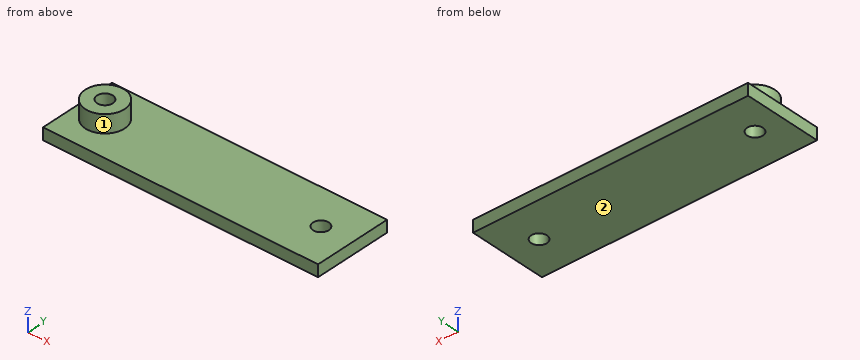
from build123d import *

# Parameters (mm, degrees)
SKETCH1_W           = 70
SKETCH1_H           = 20
BOSS_EXTRUDE1_DEPTH = 3
SKETCH2_R           = 2
CUT_EXTRUDE2_DEPTH  = 37.523964735
SKETCH3_R           = 5
BOSS_EXTRUDE2_DEPTH = 4.5
SKETCH4_R           = 2
CUT_EXTRUDE3_DEPTH  = 4.5


with BuildPart() as part:
    # Sketch1 → Boss-Extrude1 (new body)
    with BuildSketch(Plane.XY):
        Rectangle(SKETCH1_W, SKETCH1_H)
    extrude(amount=BOSS_EXTRUDE1_DEPTH)

    # Sketch2 → Cut-Extrude2 (cut, through all)
    with BuildSketch(Plane.XY.offset(3)):
        with Locations((-28, 0)):
            Circle(SKETCH2_R)
        with Locations((26.96, 0)):
            Circle(SKETCH2_R)
    extrude(amount=-CUT_EXTRUDE2_DEPTH, mode=Mode.SUBTRACT)

    # Sketch3 → Boss-Extrude2 (add)
    with BuildSketch(Plane.XY.offset(3)):
        with Locations((-28, 0)):
            Circle(SKETCH3_R)
    extrude(amount=BOSS_EXTRUDE2_DEPTH)

    # Sketch4 → Cut-Extrude3 (cut)
    with BuildSketch(Plane.XY.offset(7.5)):
        with Locations((-28, 0)):
            Circle(SKETCH4_R)
    extrude(amount=-CUT_EXTRUDE3_DEPTH, mode=Mode.SUBTRACT)


solid = part.part
Model file for the job. Use its own axes, mm. Face numbers are marked on the shaded views. A direction names the side the tool comes from. Coordinates: 2 decimals unless noted, no trailing zeros. Order: outer loops, then holes, each group sorted by start corner. A loop starts at its lowest first (then second) coordinate and runs counter-clockwise, first axis right, second up. Notation, with made-up numbers: (63, 12.25) -> (67, 12.25) arc R12 ccw to (67, 28.25) -> close; hole circle Ø10 at (-32, 29). An arc over 180 degrees is marked (long way). Return JSON: item names as keys, results as strings. Group by question number.
Item 1: Tool access for the marked faces 1 and 2: list every direction of +Z, -Z, +X, -X, +Y, -Y with a clear straight run to the whole face (end or side of a thin tool).
Item 2: Saw through at C-C on y = 0. Write the cut outline in (x, z), then the cut area to 3 significant figures.
Item 3: Saw through at B-B on z = 1.75. Write the cut outline in (x, y).
Item 4: Saw through at A-A on x = 26.96. Write the cut outline in (y, z).
Item 5: Wall check: line 1 along Y through (x, z) = (26.96, 1.85); line 2 along Y through (x, z) = (-28, 4); line 3 along Z through (x, y) = (26.5, -4.5). Give the ranges that are in metal, low to high. Write a range as [from, to].
Item 6: Saw through at D-D on x = -28. Write the cut outline in (y, z), then the cut area to 3 significant figures.
Item 7: Flat gauge pin, fed straight in: P1, Ø6, axis at x = 16.5, y = -1, coming from the +Z side. Where does the tip first touch, or does it go through?
Values found:
{
 "1": {"face 1": "+Z", "face 2": "-Z, +X, -X, +Y, -Y"},
 "2": {"outline": "(-35, 0) -> (-30, 0) -> (-30, 7.5) -> (-33, 7.5) -> (-33, 3) -> (-35, 3) -> close; (-26, 0) -> (24.96, 0) -> (24.96, 3) -> (-23, 3) -> (-23, 7.5) -> (-26, 7.5) -> close; (28.96, 0) -> (35, 0) -> (35, 3) -> (28.96, 3) -> close", "area": "213 mm2"},
 "3": {"outline": "(-35, -10) -> (35, -10) -> (35, 10) -> (-35, 10) -> close; hole circle Ø4 at (-28, 0); hole circle Ø4 at (26.96, 0)"},
 "4": {"outline": "(-10, 0) -> (-2, 0) -> (-2, 3) -> (-10, 3) -> close; (2, 0) -> (10, 0) -> (10, 3) -> (2, 3) -> close"},
 "5": {"line 1": "y = [-10, -2], [2, 10]", "line 2": "y = [-5, -2], [2, 5]", "line 3": "z = [0, 3]"},
 "6": {"outline": "(-10, 0) -> (-2, 0) -> (-2, 7.5) -> (-5, 7.5) -> (-5, 3) -> (-10, 3) -> close; (2, 0) -> (10, 0) -> (10, 3) -> (5, 3) -> (5, 7.5) -> (2, 7.5) -> close", "area": "75.0 mm2"},
 "7": {"P1": "stops at z = 3"}
}
